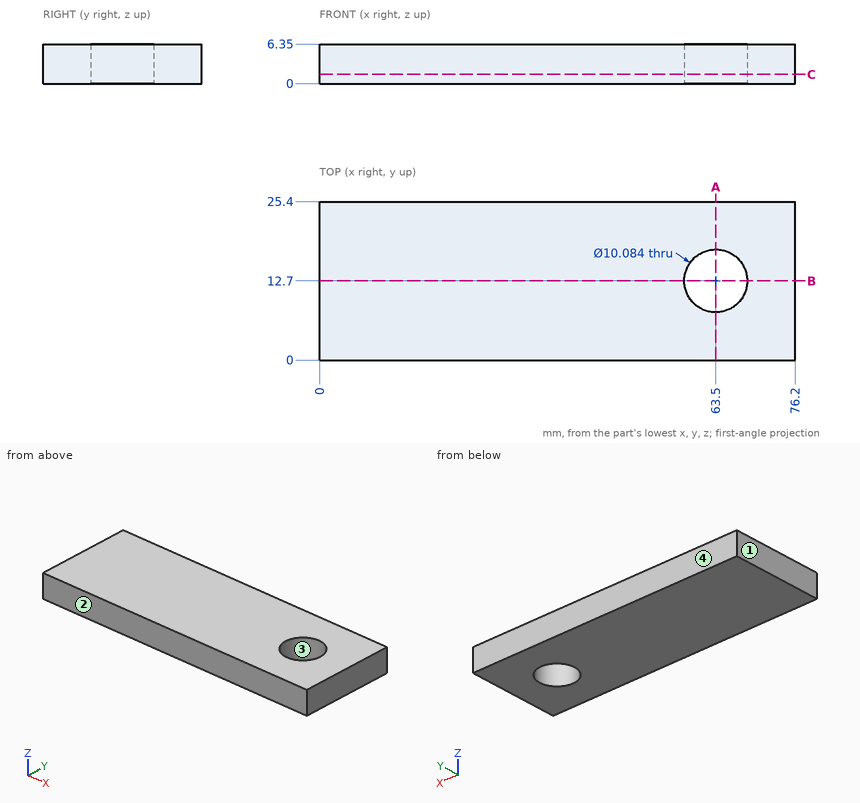
Job drawing, mm, ordinate dimensions from the low corner. One solid piece. Coordinates: 2 decimals unless noted, no trailing zeros. Write each loop counter-clockwise with the first axis right and the second up, starting at its lowest first coordinate (ties: lowest second). Pieces come first, ordered by that corner, then holes.
Item 1: Pin check, flat tip, straight feed: pin 1 (1.5 mm diameter, centred on x = 62.5, z = 4.5, fed in from -Y). Stop position of the tip, or through.
Item 2: Slice it at C-C (z = 1.5). Write the cut outline in (x, y).
Item 3: Slice it at B-B (y = 12.7). Write the cut outline in (x, z).
Item 4: Slice it at A-A (x = 63.5). Write the cut outline in (y, z).
Item 5: Probe line 1 (Y direction, x = 63.5, z = 1.5); line 2 (X direction, y = 10.5, z = 3.25). List the from-to ranges inside material, lowest first.
Item 6: Mould opens along Y. For the marked faces 1, 2, 3 and 4 say: released by +Y, released by -Y, zero draft, split by the parting line, or undercut.
Results found:
1. pin 1: stops at y = 0
2. outline: (0, 0) - (76.2, 0) - (76.2, 25.4) - (0, 25.4) - close; hole circle Ø10.08 at (63.5, 12.7)
3. outline: (0, 0) - (58.46, 0) - (58.46, 6.35) - (0, 6.35) - close; (68.54, 0) - (76.2, 0) - (76.2, 6.35) - (68.54, 6.35) - close
4. outline: (0, 0) - (7.66, 0) - (7.66, 6.35) - (0, 6.35) - close; (17.74, 0) - (25.4, 0) - (25.4, 6.35) - (17.74, 6.35) - close
5. line 1: y = 0 to 7.66, 17.74 to 25.4
5. line 2: x = 0 to 58.96, 68.04 to 76.2
6. face 1: zero draft
6. face 2: released by -Y
6. face 3: undercut
6. face 4: released by +Y
